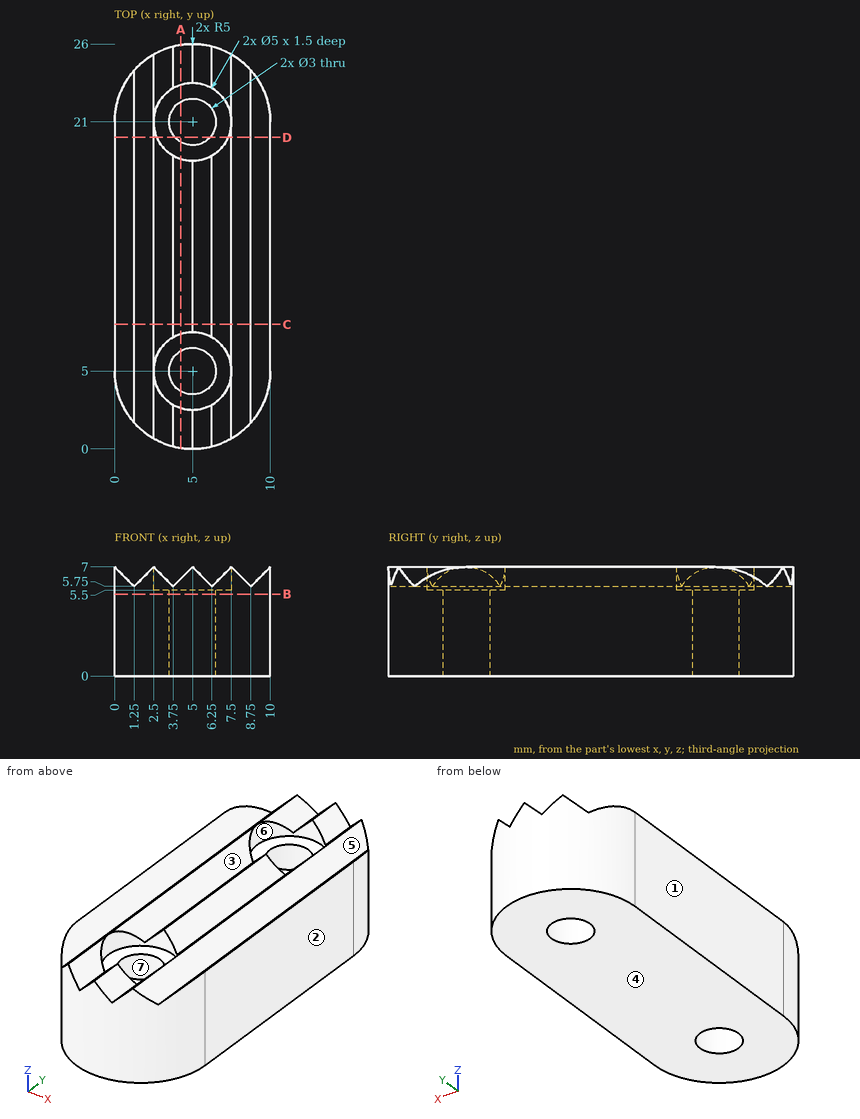
Design review of the part shown in the three views and the two pictorial views. Dimensions are in mm from the part's minimum x, y and z. A direction names the side the tool comes from. Give positions to 0.01 mm unless a question says otherwise; leave off trailing zeros. Write each loop counter-clockwise with the first axis right and the second up, starting at its lowest first coordinate (ties: lowest second). Pieces come first, ordered by that corner, then holes.
(1) Clearance check with flat-ended pins moving along their axes: pin 1 Ø6 at (x, y) = (6.5, 14) entering from +Z; pin 2 Ø1.5 at (x, y) = (6, 20.5) entering from +Z. State where each tip first meets the part, or that it passes through.
Checked values:
pin 1: stops at z = 7
pin 2: stops at z = 5.5
(2) Wall thickness on line 1 along Y through (x, z) = (5, 3.7); line 2 along Y through (x, z) = (5, 6.2); line 3 along Z through (x, y) = (1.75, 10.5): over which ranges is each line inside the solid? List them lowest first.
Checked values:
line 1: y = 0 to 3.5, 6.5 to 19.5, 22.5 to 26
line 2: y = 0 to 2.5, 7.5 to 18.5, 23.5 to 26
line 3: z = 0 to 6.25
(3) Add section C-C (y = 8). Give the boundary of the cut face in (x, z), and give its area (4 significant figures).
Checked values:
outline: (0, 0) - (10, 0) - (10, 7) - (8.75, 5.75) - (7.5, 7) - (6.25, 5.75) - (5, 7) - (3.75, 5.75) - (2.5, 7) - (1.25, 5.75) - (0, 7) - close
area: 63.75 mm2
(4) Add section A-A (x = 4.25). Give the boundary of the cut face in (y, z).
Checked values:
outline: (0.06, 0) - (3.7, 0) - (3.7, 5.5) - (2.62, 5.5) - (2.62, 6.25) - (0.06, 6.25) - close; (6.3, 0) - (19.7, 0) - (19.7, 5.5) - (18.62, 5.5) - (18.62, 6.25) - (7.38, 6.25) - (7.38, 5.5) - (6.3, 5.5) - close; (22.3, 0) - (25.94, 0) - (25.94, 6.25) - (23.38, 6.25) - (23.38, 5.5) - (22.3, 5.5) - close
(5) Add section B-B (z = 5.25). Give the boundary of the cut face in (x, y).
Checked values:
outline: (0, 5) arc R5 ccw to (10, 5) - (10, 21) arc R5 ccw to (0, 21) - close; hole circle Ø3 at (5, 5); hole circle Ø3 at (5, 21)
(6) Mouldability with a two-part tool opening along X and no side actions: class the marked faces 1, 2, 3 and 4 as +X half, -X half, draft (parallel to the pull), parting line (faces both ways), or undercut.
Checked values:
face 1: -X half
face 2: +X half
face 3: undercut
face 4: draft
(7) Tool access review of the marked faces 5, 6 and 7: name each direction out of +Z, -Z, +X, -X, +Y, -Y from which nothing blocks a thin tool from reaching the whole face with its end or side.
Checked values:
face 5: +Z, +Y, -Y
face 6: +Z
face 7: +Z, -Z
(8) Add section D-D (y = 20). Give the boundary of the cut face in (x, z).
Checked values:
outline: (0, 0) - (3.88, 0) - (3.88, 5.5) - (2.71, 5.5) - (2.71, 6.79) - (2.5, 7) - (1.25, 5.75) - (0, 7) - close; (6.12, 0) - (10, 0) - (10, 7) - (8.75, 5.75) - (7.5, 7) - (7.29, 6.79) - (7.29, 5.5) - (6.12, 5.5) - close
